Build history of the part. All positions in model axes, mm. Face numbers are marked on the shaded views. A direction names the side the tool comes from. Coordinates: 2 decimals unless noted, no trailing zeros. Order: outer loops, then holes, each group sorted by start corner. A loop starts at its lowest first (then second) coordinate and runs counter-clockwise, first axis right, second up. Notation, with made-up numbers: (73, 30) -> (106, 30) arc R10 ccw to (106, 41) -> close; hole circle Ø10 at (68.25, 82). An arc over 180 degrees is marked (long way). Write each question's results on one line, items separated by ' | '.
from build123d import *

# Parameters (mm, degrees)
EXTRUDE_1_DEPTH     = 3
SKETCH_2_R          = 1.65
CUT_EXTRUDE_1_DEPTH = 3
FILLET_2_R          = 5
SKETCH_3_W          = 44.5
SKETCH_3_H          = 15.05
CUT_EXTRUDE_2_DEPTH = 0.5


with BuildPart() as part:
    # ｽｹｯﾁ1 → ﾎﾞｽ - 押し出し1 (new body)
    with BuildSketch(Plane.XY):
        Polygon((-11.490666647, 9.641814145), (0, 0), (2.5, -2.097749078), (2.5, -16), (45, -16), (45, 0), (28.925442436, 34.47199994), (17.434775789, 44.113814086), align=None)
    extrude(amount=EXTRUDE_1_DEPTH)

    # ｽｹｯﾁ2 → ｶｯﾄ - 押し出し1 (cut)
    with BuildSketch(Plane.XY.offset(3)):
        with Locations((7.5, -8.5)):
            Circle(SKETCH_2_R)
        with Locations((-0.924426251, 10.566240396)):
            Circle(SKETCH_2_R)
        with Locations((18.35920204, 33.54757369)):
            Circle(SKETCH_2_R)
        with Locations((37.5, -8.5)):
            Circle(SKETCH_2_R)
    extrude(amount=-CUT_EXTRUDE_1_DEPTH, mode=Mode.SUBTRACT)

    # ﾌｨﾚｯﾄ2
    fillet_2_edges = [part.edges().sort_by_distance(p)[0] for p in [
        (-11.490666647, 9.641814145, 1.5),
        (17.434775789, 44.113814086, 1.5),
        (28.925442436, 34.47199994, 1.5),
        (45, 0, 1.5),
        (45, -16, 1.5),
        (2.5, -16, 1.5),
        (2.5, -2.097749078, 1.5),
    ]]
    fillet(fillet_2_edges, radius=FILLET_2_R)

    # ｽｹｯﾁ3 → ｶｯﾄ - 押し出し2 (cut)
    with BuildSketch(Plane.XY.offset(3)):
        Polygon((17.434775789, 44.113814086), (-12.133454256, 8.875769702), (-0.604485388, -0.798183824), (28.963744658, 34.43986056), align=None)
        with Locations((22.75, -8.475)):
            Rectangle(SKETCH_3_W, SKETCH_3_H)
    extrude(amount=-CUT_EXTRUDE_2_DEPTH, mode=Mode.SUBTRACT)


solid = part.part
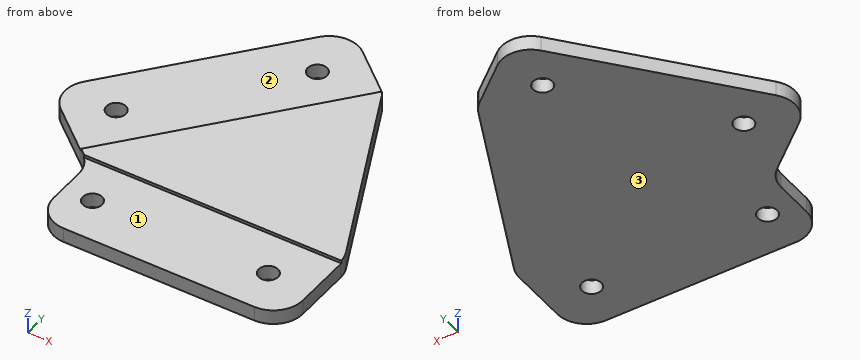
Item 1: Tool access for the marked faces 1, 2 and 3: list every direction of +Z, -Z, +X, -X, +Y, -Y with a clear straight run to the whole face (end or side of a thin tool).
Answer:
face 1: +Z, +X, -X, -Y | face 2: +Z, -X, +Y | face 3: -Z, +X, -X, +Y, -Y
Item 2: Slice it at A-A, the plane y = -8.5. List the corners of the cut face in (x, z), and give its area (4 significant figures).
Answer:
outline: (2.5, 0) -> (5.85, 0) -> (5.85, 2.5) -> (2.5, 2.5) -> close; (9.15, 0) -> (35.85, 0) -> (35.85, 2.5) -> (9.15, 2.5) -> close; (39.15, 0) -> (45, 0) -> (45, 2.5) -> (39.15, 2.5) -> close | area: 89.75 mm^2
Item 3: Pin check, flat tips, straight feed: pin 1 (3 mm diameter, centred on x = 18.36, y = 33.55, fed in from +Z) (3 decimals); pin 2 (4.5 mm diameter, centred on x = 37.5, y = -8.5, fed in from +Z); pin 3 (1 mm diameter, centred on y = 25.5, z = 0.5, fed in from -X); pin 4 (1.2 mm diameter, centred on y = -7, z = 1, fed in from -X). Stop position of each tip, or through.
Answer:
pin 1: passes through | pin 2: stops at z = 2.5 | pin 3: stops at x = 1.4 | pin 4: stops at x = 2.5
Item 4: Slice it at D-D, the plane x = 12. List the corners of the cut face in (y, z), and give its area (3 significant figures).
Answer:
outline: (-16, 0) -> (37.64, 0) -> (37.64, 2.5) -> (14.22, 2.5) -> (14.22, 3) -> (-0.95, 3) -> (-0.95, 2.5) -> (-16, 2.5) -> close | area: 142 mm^2
Item 5: Slice it at C-C, the plane z = 1.55. State how many separate pieces and enclosed holes the cut face has, and give its area (3 significant figures).
Answer:
separate pieces: 1 | enclosed holes: 4 | area: 2,080 mm^2
Item 6: Slice it at B-B, the plane x = 37.5. List the corners of the cut face in (y, z).
Answer:
outline: (-16, 0) -> (-10.15, 0) -> (-10.15, 2.5) -> (-16, 2.5) -> close; (-6.85, 0) -> (16.08, 0) -> (16.08, 3) -> (-0.95, 3) -> (-0.95, 2.5) -> (-6.85, 2.5) -> close
Item 7: Drill centre lines: line 1 (X direction, y = -10, z = 0.9); line 2 (Z direction, x = 11, y = 25.5); line 3 (X direction, y = 34, z = 0.5). Where is each one in solid material? Low to high. Write a range as from..to.
Answer:
line 1: x = 2.5..6.81, 8.19..36.81, 38.19..45 | line 2: z = 0..2.5 | line 3: x = 8.95..16.77, 19.95..29.11
